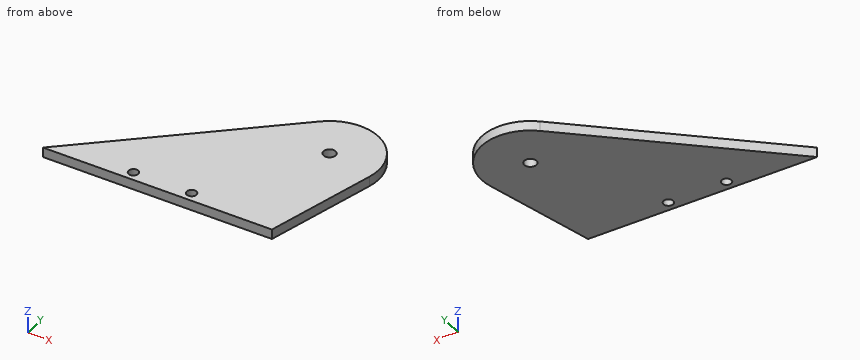
from build123d import *

# Parameters (mm, degrees)
SKETCH_1_R      = 1.25
SKETCH_1_R_2    = 1
EXTRUDE_1_DEPTH = 2


with BuildPart() as part:
    # 草圖1 → 填料-伸長1 (new body)
    with BuildSketch(Plane.XY):
        with BuildLine():
            Line((-41.078680873, -25.246867961), (3.125001345, -25.246867961))
            Line((3.125001345, -25.246867961), (4.118524153, -25.246867961))
            Line((4.118524153, -25.246867961), (9.71355395, -2.376314303))
            ThreePointArc((9.71355395, -2.376314303), (5.139430957, 8.578242795), (-6.677431122, 7.443917894))
            Line((-6.677431122, 7.443917894), (-43.120716176, -25.246867961))
            Line((-43.120716176, -25.246867961), (-41.078680873, -25.246867961))
        make_face()
        Circle(SKETCH_1_R, mode=Mode.SUBTRACT)
        with Locations((-25.732609449, -23.246867961)):
            Circle(SKETCH_1_R_2, mode=Mode.SUBTRACT)
        with Locations((-13.732609449, -23.246867961)):
            Circle(SKETCH_1_R_2, mode=Mode.SUBTRACT)
    extrude(amount=EXTRUDE_1_DEPTH)


solid = part.part
The listing builds one solid part. Answer for the finished solid, in the listing's coordinates (mm). Coordinates: 2 decimals unless noted, no trailing zeros. Order: outer loops, then holes, each group sorted by start corner. A loop starts at its lowest first (then second) coordinate and runs counter-clockwise, first axis right, second up. Notation, with made-up numbers: (-31, 55) -> (5, 55) arc R16 ccw to (5, 66) -> close; hole circle Ø10 at (49, -22.5). An arc over 180 degrees is marked (long way). Answer in a Markdown table with one row per item. Add a question column.
Item 1: Find section A-A (x = 0). Write down the section's boundary in (y, z), then the cut area to 3 significant figures.
Item 2: Find section C-C (z = 0.7). Write down the section's boundary in (x, y).
Item 3: Find the intervals of material crossed by L1, parallel to Y at x = 0, z = 1.15; L2, parallel to X at y = -23, z = 1.9; L3, parallel to X at y = -1, z = 1.1, in increasing order. Write a range as from..to.
Item 4: Find section D-D (y = -9.5). Write down the section's boundary in (x, z).
Item 5: Find section B-B (y = 0). Write down the section's boundary in (x, z).
Item 6: This flat-tipped pin is pushed along its axis until it touches: P1, Ø1.8, axis at x = -13.73, y = -23.25, coming from the +Z side. Where does it stop, or does it pass through?
Result set:
| question | item | result |
|---|---|---|
| 1 | outline | (-25.25, 0) -> (-1.25, 0) -> (-1.25, 2) -> (-25.25, 2) -> close; (1.25, 0) -> (10, 0) -> (10, 2) -> (1.25, 2) -> close |
| 1 | area | 65.5 mm² |
| 2 | outline | (-43.12, -25.25) -> (4.12, -25.25) -> (9.71, -2.38) arc R10 ccw to (-6.68, 7.44) -> close; hole circle Ø2 at (-25.73, -23.25); hole circle Ø2 at (-13.73, -23.25); hole circle Ø2.5 at (0, 0) |
| 3 | L1 | y = -25.25..-1.25, 1.25..10 |
| 3 | L2 | x = -40.62..-26.7, -24.76..-14.7, -12.76..4.67 |
| 3 | L3 | x = -16.09..-0.75, 0.75..9.95 |
| 4 | outline | (-25.57, 0) -> (7.97, 0) -> (7.97, 2) -> (-25.57, 2) -> close |
| 5 | outline | (-14.98, 0) -> (-1.25, 0) -> (-1.25, 2) -> (-14.98, 2) -> close; (1.25, 0) -> (10, 0) -> (10, 2) -> (1.25, 2) -> close |
| 6 | P1 | passes through |
